Could you check a few things on this model? Use its own coordinates, in mm. A direction names the side the tool comes from. Round coordinates to 2 decimals unless told otherwise and drop trailing zeros. Order: outer loops, then holes, each group sorted by start corner. A loop starts at its lowest first (then second) coordinate and runs counter-clockwise, first axis right, second up. Notation, with made-up numbers: (13.5, 64.5) -> (23.5, 64.5) arc R31 ccw to (23.5, 99.5) -> close; hole circle Ø9 at (-15.75, 49). An arc over 180 degrees is marked (long way). One line per question, with ' | ' between items.
```python
from build123d import *

# Parameters (mm, degrees)
F0_R     = 10.95
F1_DEPTH = 7


# Not quite as in the source:
# - a feature names something its author has since deleted; it is built from what else it names


with BuildPart() as f1:
    # F0 (on Top) → F1 (new body)
    with BuildSketch(Plane.XY):
        with BuildLine():
            ThreePointArc((-56.191941013, 7.2029190708), (-65.7378825591, -15.8430224752), (-42.691941013, -6.2970809292))
            ThreePointArc((-42.691941013, -6.2970809292), (-46.645999467, 3.2488606168), (-56.191941013, 7.2029190708))
        make_face()
        with Locations((-56.191941013, -6.2970809292)):
            Circle(F0_R, mode=Mode.SUBTRACT)
        with BuildLine():
            Line((-42.691941013, -6.2970809292), (-26.191941013, -6.2970809292))
            ThreePointArc((-26.191941013, -6.2970809292), (-38.5028813329, 1.6629959269), (-36.295891117, 16.156141524))
            Line((-36.295891117, 16.156141524), (-56.191941013, 7.2029190708))
            ThreePointArc((-56.191941013, 7.2029190708), (-46.645999467, 3.2488606168), (-42.691941013, -6.2970809292))
        make_face()
        with BuildLine():
            ThreePointArc((-20.4170961141, -4.9995874911), (-14.7855742353, -0.0182163615), (-12.691941013, 7.2029190708))
            ThreePointArc((-12.691941013, 7.2029190708), (-14.704995322, 14.295173909), (-20.1438045227, 19.2723036862))
            Line((-20.1438045227, 19.2723036862), (-26.191941013, 20.7029190708))
            Line((-26.191941013, 20.7029190708), (-36.295891117, 16.156141524))
            ThreePointArc((-36.295891117, 16.156141524), (-38.5028813329, 1.6629959269), (-26.191941013, -6.2970809292))
            Line((-26.191941013, -6.2970809292), (-20.4170961141, -4.9995874911))
        make_face()
        with Locations((-26.191941013, 7.2029190708)):
            Circle(F0_R, mode=Mode.SUBTRACT)
        with BuildLine():
            ThreePointArc((-20.1438045227, 19.2723036862), (-14.704995322, 14.295173909), (-12.691941013, 7.2029190708))
            ThreePointArc((-12.691941013, 7.2029190708), (-14.7855742353, -0.0182163615), (-20.4170961141, -4.9995874911))
            Line((-20.4170961141, -4.9995874911), (3.0783548298, 0.27937566))
            ThreePointArc((3.0783548298, 0.27937566), (-7.5094084371, 5.4038596161), (-10.0591238534, 16.8868913633))
            Line((-10.0591238534, 16.8868913633), (-20.1438045227, 19.2723036862))
        make_face()
        with BuildLine():
            ThreePointArc((16.5783548298, 13.77937566), (4.6426498429, 27.1884390543), (-10.0591238534, 16.8868913633))
            ThreePointArc((-10.0591238534, 16.8868913633), (-7.5094084371, 5.4038596161), (3.0783548298, 0.27937566))
            ThreePointArc((3.0783548298, 0.27937566), (12.6242963759, 4.233434114), (16.5783548298, 13.77937566))
        make_face()
        with BuildLine():
            ThreePointArc((14.0283548298, 13.77937566), (1.8095377637, 2.9031353513), (-7.5776001022, 16.2999161749))
            ThreePointArc((-7.5776001022, 16.2999161749), (4.347171896, 24.6556159687), (14.0283548298, 13.77937566))
        make_face(mode=Mode.SUBTRACT)
    extrude(amount=F1_DEPTH)


solid = f1.part
```
1. I want a section at B-B on y = -2.5. List the corners of the cut face in (x, z) for me.
From the geometry:
outline: (-69.15, 0) -> (-66.46, 0) -> (-66.46, 7) -> (-69.15, 7) -> close; (-45.92, 0) -> (-31.27, 0) -> (-31.27, 7) -> (-45.92, 7) -> close; (-21.12, 0) -> (-9.29, 0) -> (-9.29, 7) -> (-21.12, 7) -> close
2. On a 3-axis mill with a long thin cutter (end or side, diameter ignored), from which of +Z, -Z, +X, -X, +Y, -Y can I reach the whole of each face in a straight line? I mean faces 4 (the face through (-35, -6.297, 3)), 5 (the face through (-34.88, 0.54, 3.45)). Say none if no direction works.
From the geometry:
face 4: +Z, -Z, +X, -Y | face 5: +Z, -Z
3. I want a section at C-C on y = -12. List the corners of the cut face in (x, z) for me.
From the geometry:
outline: (-68.43, 0) -> (-65.54, 0) -> (-65.54, 7) -> (-68.43, 7) -> close; (-46.84, 0) -> (-43.96, 0) -> (-43.96, 7) -> (-46.84, 7) -> close
4. If we mould it in two halves opening along X, with no side actions, what happens to faces 1 (the face through (-27, -5, 7)), 2 (the face through (-40.98, 14.05, 3.45)), 3 (the face through (10.001, 5.295, 3.451))? For each: pulls with the +X half, pulls with the -X half, needs draft (parallel to the pull), parting line crosses it, or undercut.
From the geometry:
face 1: needs draft | face 2: pulls with the -X half | face 3: undercut
5. I want a section at D-D on z = 5.25. List the corners of the cut face in (x, y) for me.
From the geometry:
outline: (-56.19, 7.2) arc R13.5 ccw (long way) to (-42.69, -6.3) -> (-26.19, -6.3) -> (3.08, 0.28) arc R13.5 ccw (long way) to (-10.06, 16.89) -> (-26.19, 20.7) -> close; hole circle Ø21.9 at (-56.19, -6.3); hole circle Ø21.9 at (-26.19, 7.2); hole circle Ø21.9 at (3.08, 13.78)
6. I need wall thicknesses on probe 1 along X at (y, z) = (5, 3.5); probe 2 along X at (y, z) = (11, 4); probe 3 along Y at (x, z) = (-34.5, 3.25). Which ranges of each line are inside material? Lowest first, please.
From the geometry:
probe 1: x = -63.58 to -36.92, -15.47 to -3.47, 9.62 to 13.33 | probe 2: x = -47.75 to -36.46, -15.92 to -7.51, 13.67 to 16.29 | probe 3: y = -6.3 to 0.07, 14.34 to 16.96
7. I want a section at A-A on x = -47. List the corners of the cut face in (y, z) for me.
From the geometry:
outline: (-16.18, 0) -> (-12.25, 0) -> (-12.25, 7) -> (-16.18, 7) -> close; (-0.35, 0) -> (11.34, 0) -> (11.34, 7) -> (-0.35, 7) -> close
8. I'm going to push flat-ended pins straight in: pin 1 (10 mm diameter, centred on x = -52, y = 3, fed in from -Z); pin 2 (1 mm diameter, centred on x = -25, z = 3, fed in from +Y); pin 3 (2 mm diameter, centred on x = -17, y = 10.5, fed in from +Z); pin 4 (1.5 mm diameter, centred on y = 0.5, z = 5, fed in from +X). Where does each tip first touch, or does it pass through?
From the geometry:
pin 1: stops at z = 0 | pin 2: stops at y = 20.54 | pin 3: passes through | pin 4: stops at x = 8.1
